The listing builds one solid part. Answer for the finished solid, in the listing's coordinates (mm). Give positions to 0.01 mm unless a question says otherwise; leave off trailing zeros. Write each loop counter-clockwise with the first axis right and the second up, starting at its lowest first coordinate (ties: lowest second). Pieces come first, ordered by that corner, then holes. Notation, with made-up numbers: (15.25, 39) - (33.25, 39) arc R25 ccw to (33.25, 58) - close; hole circle Ø10 at (-12, 17.5). An arc over 180 degrees is marked (long way). One line per question, with ' | ' between items. Start each with the question number.
1. A cutting plane is placed at C-C (x = 48). Determine the outline of the cut face in (y, z).
2. A cutting plane is placed at D-D (z = 4). Determine the outline of the cut face in (x, y), then the cut area to 3 significant figures.
3. Given P1, Ø1.5, axis at y = 1.5, z = -15, coming from the -X side; P2, Ø1.5, axis at y = 3, z = -26, coming from the +X side, each flat-ended and moving along its own axis, determine where each tip first touches the part or whether it passes through.
4. A cutting plane is placed at B-B (z = -24). Determine the outline of the cut face in (x, y), then the cut area to 3 significant figures.
5. Find the intervals of material crossed by L1, parallel to X at y = 2.9, z = -4; L2, parallel to X at y = 1.65, z = -6; L3, parallel to Z at x = 23.5, y = 3.55, in increasing order. Write a range as from..to.
6. A cutting plane is placed at A-A (x = 6). Determine the outline of the cut face in (y, z).
```python
from build123d import *

# Parameters (mm, degrees)
SKETCH_1_W      = 80
SKETCH_1_H      = 20
SKETCH_1_R      = 1
SKETCH_1_W_2    = 23
SKETCH_1_H_2    = 12
SKETCH_1_R_2    = 1.5
EXTRUDE_1_DEPTH = 4
FILLET_1_R      = 3
SKETCH_2_W      = 10
SKETCH_2_H      = 24
SKETCH_2_R      = 1.5
EXTRUDE_2_DEPTH = 4
FILLET_2_R      = 10
FILLET_3_R      = 2


with BuildPart() as part:
    # 草图1 → 凸台-拉伸1 (new body)
    # profile 1 of 3: a face of its own
    with BuildSketch(Plane(origin=(0, 0, 0), x_dir=(1, 0, 0), z_dir=(0, 1, 0))):
        Rectangle(SKETCH_1_W, SKETCH_1_H)
        with Locations(Location((-36, -4, 0), (0, 0, 270))):
            Circle(SKETCH_1_R, mode=Mode.SUBTRACT)
        with Locations(Location((-24, -4, 0), (0, 0, 270))):
            Circle(SKETCH_1_R, mode=Mode.SUBTRACT)
        with Locations(Location((36, 4, 0), (0, 0, 270))):
            Circle(SKETCH_1_R, mode=Mode.SUBTRACT)
        with Locations(Location((24, 4, 0), (0, 0, 270))):
            Circle(SKETCH_1_R, mode=Mode.SUBTRACT)
        with Locations(Location((14, 6, 0), (0, 0, 270))):
            Circle(SKETCH_1_R, mode=Mode.SUBTRACT)
        with Locations(Location((6, 6, 0), (0, 0, 270))):
            Circle(SKETCH_1_R, mode=Mode.SUBTRACT)
        with Locations(Location((14, -6, 0), (0, 0, 270))):
            Circle(SKETCH_1_R, mode=Mode.SUBTRACT)
        with Locations(Location((6, -6, 0), (0, 0, 270))):
            Circle(SKETCH_1_R, mode=Mode.SUBTRACT)
        with Locations(Location((36, -4, 0), (0, 0, 270))):
            Circle(SKETCH_1_R, mode=Mode.SUBTRACT)
        with Locations(Location((24, -4, 0), (0, 0, 270))):
            Circle(SKETCH_1_R, mode=Mode.SUBTRACT)
        with Locations(Location((-36, 4, 0), (0, 0, 270))):
            Circle(SKETCH_1_R, mode=Mode.SUBTRACT)
        with Locations(Location((-24, 4, 0), (0, 0, 270))):
            Circle(SKETCH_1_R, mode=Mode.SUBTRACT)
    # profile 2 of 3: a face of its own
    with BuildSketch(Plane(origin=(0, 0, 0), x_dir=(1, 0, 0), z_dir=(0, 1, 0))):
        with Locations((51.5, 0)):
            Rectangle(SKETCH_1_W_2, SKETCH_1_H)
        with Locations(Location((46, -6, 0), (0, 0, 270))):
            Circle(SKETCH_1_R, mode=Mode.SUBTRACT)
        with Locations(Location((46, 6, 0), (0, 0, 270))):
            Circle(SKETCH_1_R, mode=Mode.SUBTRACT)
        with Locations(Location((54, -6, 0), (0, 0, 270))):
            Circle(SKETCH_1_R, mode=Mode.SUBTRACT)
        with Locations(Location((54, 6, 0), (0, 0, 270))):
            Circle(SKETCH_1_R, mode=Mode.SUBTRACT)
    # profile 3 of 3: a face of its own
    with BuildSketch(Plane(origin=(0, 0, 0), x_dir=(1, 0, 0), z_dir=(0, 1, 0))):
        with Locations((51.5, 16)):
            Rectangle(SKETCH_1_W_2, SKETCH_1_H_2)
        with Locations(Location((56, 18, 0), (0, 0, 270))):
            Circle(SKETCH_1_R_2, mode=Mode.SUBTRACT)
        with Locations(Location((48, 18, 0), (0, 0, 270))):
            Circle(SKETCH_1_R_2, mode=Mode.SUBTRACT)
    extrude(amount=EXTRUDE_1_DEPTH)

    # 圆角1
    fillet_1_edges = [part.edges().sort_by_distance(p)[0] for p in [
        (-40, 2, 10),
        (-40, 2, -10),
        (40, 2, -10),
        (40, 2, -22),
        (63, 2, -22),
        (63, 2, 10),
    ]]
    fillet(fillet_1_edges, radius=FILLET_1_R)

    # 草图2 → 凸台-拉伸2 (add)
    with BuildSketch(Plane(origin=(0, 4, 0), x_dir=(1, 0, 0), z_dir=(0, 1, 0))):
        with Locations((13, 22)):
            Rectangle(SKETCH_2_W, SKETCH_2_H)
        with Locations(Location((13, 24, 0), (0, 0, 270))):
            Circle(SKETCH_2_R, mode=Mode.SUBTRACT)
        with Locations(Location((13, 16, 0), (0, 0, 270))):
            Circle(SKETCH_2_R, mode=Mode.SUBTRACT)
    extrude(amount=-EXTRUDE_2_DEPTH)

    # 圆角2
    fillet_2_edges = [part.edges().sort_by_distance(p)[0] for p in [
        (18, 2, -10),
        (8, 2, -10),
    ]]
    fillet(fillet_2_edges, radius=FILLET_2_R)

    # 圆角3
    fillet_3_edges = [part.edges().sort_by_distance(p)[0] for p in [
        (8, 2, -34),
        (18, 2, -34),
    ]]
    fillet(fillet_3_edges, radius=FILLET_3_R)


solid = part.part
```
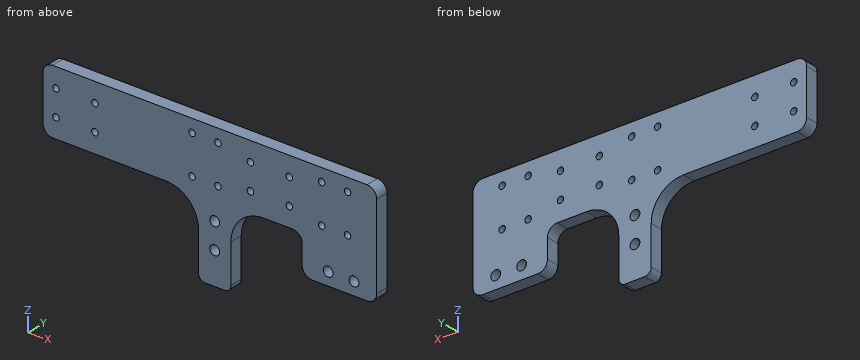
Determined:
1) outline: (0, -22) - (4, -22) - (4, -19.5) - (0, -19.5) - close; (0, -16.5) - (4, -16.5) - (4, 10) - (0, 10) - close
2) outline: (-40, 0) - (-37, 0) - (-37, 4) - (-40, 4) - close; (-35, 0) - (-25, 0) - (-25, 4) - (-35, 4) - close; (-23, 0) - (23, 0) - (23, 4) - (-23, 4) - close; (25, 0) - (35, 0) - (35, 4) - (25, 4) - close; (37, 0) - (63, 0) - (63, 4) - (37, 4) - close | area: 380 mm2
3) P1: x = 6.18 | P2: x = 18
4) outline: (8, 0) - (11.5, 0) - (11.5, 4) - (8, 4) - close; (14.5, 0) - (18, 0) - (18, 4) - (14.5, 4) - close | area: 28.0 mm2
5) L1: -40..-37, -35..-25, -23..23, 25..35, 37..63 | L2: -40..5, 7..13, 15..45, 47..53, 55..63 | L3: -11.07..-4.87, -3.13..3.13, 4.87..10
6) outline: (0, -14) - (4, -14) - (4, -7) - (0, -7) - close; (0, -5) - (4, -5) - (4, 5) - (0, 5) - close; (0, 7) - (4, 7) - (4, 10) - (0, 10) - close
